```python
from build123d import *

# Parameters (mm, degrees)
SKETCH027_W     = 18
SKETCH027_H     = 25
SKETCH027_R     = 1.6
PAD008_DEPTH    = 4
SKETCH028_R     = 1.5
CHAMFER011_SIZE = 1
CHAMFER033_SIZE = 1
CHAMFER039_SIZE = 0.4


with BuildPart() as part:
    # Sketch027 (on Binder) → Pad008 (new body)
    with BuildSketch(Plane.XY):
        with Locations((-28.5, 0)):
            Rectangle(SKETCH027_W, SKETCH027_H)
        with Locations((-28.5, 7.5)):
            Circle(SKETCH027_R, mode=Mode.SUBTRACT)
        with Locations((-28.5, -7.5)):
            Circle(SKETCH027_R, mode=Mode.SUBTRACT)
    extrude(amount=PAD008_DEPTH)

    # Pipe002: sweep along a path in Sketch029
    with BuildLine(Plane(origin=(0, 0, 0), x_dir=(1, 0, 0), z_dir=(0, 0, -1))) as pipe002_path:
        Line((-37.5, 0), (-32.5, 0))
        ThreePointArc((-32.5, 0), (-25.713288, 0.99695), (-19.5, 3.903567))
        Line((-19.5, 3.903567), (0, 16.774801))
    # Sketch028 (on Face4 of Pad008) → Pipe002 (sweep, cut)
    with BuildSketch(Plane(origin=(-37.5, 0, 0), x_dir=(0, -1, 0), z_dir=(-1, 0, 0))):
        Circle(SKETCH028_R)
    sweep(path=pipe002_path.line, mode=Mode.SUBTRACT)

    # Chamfer011
    chamfer011_edges = [part.edges().sort_by_distance(p)[0] for p in [
        (-37.5, 0, 1.5),
        (-19.5, -2.700188, 1.106038),
    ]]
    chamfer(chamfer011_edges, length=CHAMFER011_SIZE)

    # Chamfer033
    chamfer033_edges = [part.edges().sort_by_distance(p)[0] for p in [
        (-37.5, -12.5, 2),
        (-19.5, -12.5, 2),
        (-19.5, 12.5, 2),
        (-37.5, 12.5, 2),
    ]]
    chamfer(chamfer033_edges, length=CHAMFER033_SIZE)

    # Chamfer039
    chamfer039_edges = [part.edges().sort_by_distance(p)[0] for p in [
        (-28.5, 12.5, 4),
        (-37, 12, 4),
        (-20, 12, 4),
        (-37.5, 0, 4),
        (-19.5, 0, 4),
        (-37, -12, 4),
        (-20, -12, 4),
        (-28.5, -12.5, 4),
        (-30.1, 7.5, 4),
        (-30.1, -7.5, 4),
    ]]
    chamfer(chamfer039_edges, length=CHAMFER039_SIZE)


with BuildPart() as part_1:
    # Body005 placement: moved
    add(part.part.moved(Location((0, 0, 3.5))))


solid = part_1.part
```
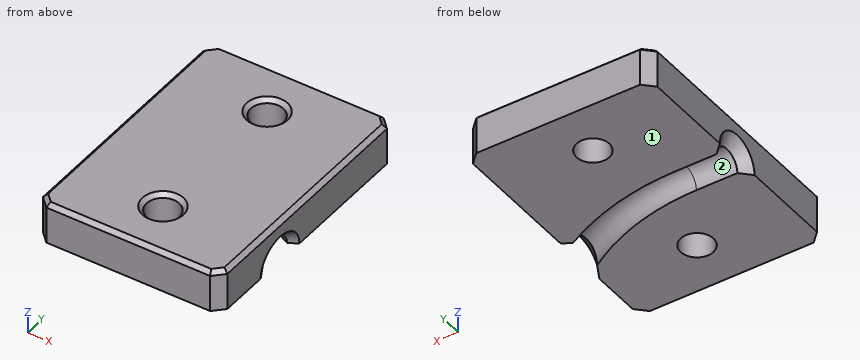
Input: part model. Units: mm. Frame: model coordinates. Face numbers are marked on the shaded views. A direction names the side the tool comes from. Round coordinates to 2 decimals unless told otherwise and drop trailing zeros. Write each loop counter-clockwise with the first axis right and the second up, starting at its lowest first coordinate (ties: lowest second). Pieces come first, ordered by that corner, then holes. Notation, with made-up numbers: (65, -29.75) - (85, -29.75) arc R4 ccw to (85, -23.75) - close; hole circle Ø8 at (80.5, 69.5). An arc over 180 degrees is marked (long way). Write item = value, one per line.
(1) Contact query for flat-ended pins moving along their axis: pin 1 Ø1.9 at (x, y) = (-28.5, -7.5) entering from +Z; pin 2 Ø3.5 at (x, y) = (-28.5, 7.5) entering from -Z. Output: stop coordinate, or through.
Geometry check:
pin_1 = through
pin_2 = 3.5
(2) Section query B-B on z = 6.55. Output: boundary loops of the cut face in (x, y).
Geometry check:
outline = (-37.5, -11.5) - (-36.5, -12.5) - (-20.5, -12.5) - (-19.5, -11.5) - (-19.5, 11.5) - (-20.5, 12.5) - (-36.5, 12.5) - (-37.5, 11.5) - close; hole circle Ø3.2 at (-28.5, -7.5); hole circle Ø3.2 at (-28.5, 7.5)
(3) Section query C-C on x = -33.25. Output: boundary loops of the cut face in (y, z).
Geometry check:
outline = (-12.5, 3.5) - (-1.5, 3.5) arc R1.5 cw to (1.5, 3.5) - (12.5, 3.5) - (12.5, 7.1) - (12.1, 7.5) - (-12.1, 7.5) - (-12.5, 7.1) - close
(4) Material intervals for probe 1 along Y at (x, z) = (-28.5, 5.45); probe 2 along Y at (x, z) = (-29.5, 5.3); probe 3 along Y at (x, z) = (-28, 4), sorted ascending.
Geometry check:
probe_1 = -12.5 to -9.1, -5.9 to 5.9, 9.1 to 12.5
probe_2 = -12.5 to -8.75, -6.25 to 6.25, 8.75 to 12.5
probe_3 = -12.5 to -9.02, -5.98 to -1.88, 1.01 to 5.98, 9.02 to 12.5
(5) Section query D-D on z = 4.75. State how many separate pieces and enclosed holes the cut face has, then the cut area to 3 significant figures.
Geometry check:
separate_pieces = 2
enclosed_holes = 2
area = 398 mm^2
(6) Section query A-A on y = 7.5. Output: boundary loops of the cut face in (x, z).
Geometry check:
outline = (-37.5, 3.5) - (-30.1, 3.5) - (-30.1, 7.1) - (-30.5, 7.5) - (-37.1, 7.5) - (-37.5, 7.1) - close; (-26.9, 3.5) - (-19.5, 3.5) - (-19.5, 7.1) - (-19.9, 7.5) - (-26.5, 7.5) - (-26.9, 7.1) - close
(7) Access query for the marked faces 1 and 2. Directions: +Z, -Z, +X, -X, +Y, -Y. A direction counts if a zero-diameter tool reaches every point of the face in a straight line with its end or side. Return the directions, or none.
Geometry check:
face_1 = -Z, +X, -X, +Y, -Y
face_2 = -Z, -X
